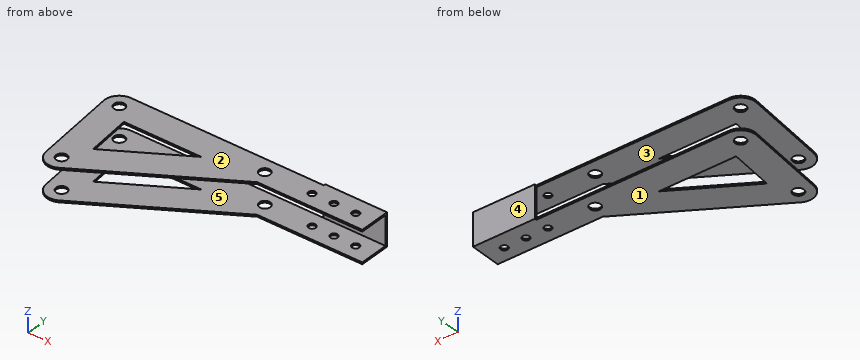
```python
from build123d import *

# Parameters (mm, degrees)
SKETCH_1_R      = 1.5
SKETCH_1_R_2    = 1
EXTRUDE_1_DEPTH = 0.5
SKETCH_2_R      = 1.5
SKETCH_2_R_2    = 1
EXTRUDE_2_DEPTH = 0.5
SKETCH_3_W      = 17
SKETCH_3_H      = 9
EXTRUDE_3_DEPTH = 0.5


with BuildPart() as part:
    # Sketch 1 → Extrude 1 (new body)
    with BuildSketch(Plane.XY):
        with BuildLine():
            Line((-6.593488685, 7.462066188), (63.406511315, 7.462066188))
            Line((63.406511315, 7.462066188), (63.406511315, -0.537933812))
            Line((63.406511315, -0.537933812), (34.527914712, -0.537933812))
            Line((34.527914712, -0.537933812), (-2.101613692, -22.82810419))
            ThreePointArc((-2.101613692, -22.82810419), (-5.955067108, -22.996117417), (-8.158923454, -19.830623953))
            Line((-8.158923454, -19.830623953), (-10.571423454, 3.04250097))
            ThreePointArc((-10.571423454, 3.04250097), (-9.566556198, 6.138046301), (-6.593488685, 7.462066188))
        make_face()
        with Locations((-6.593488685, 3.462066188)):
            Circle(SKETCH_1_R, mode=Mode.SUBTRACT)
        with Locations((33.406511315, 3.462066188)):
            Circle(SKETCH_1_R, mode=Mode.SUBTRACT)
        with Locations((-4.180988685, -19.411058735)):
            Circle(SKETCH_1_R, mode=Mode.SUBTRACT)
        with Locations((58.406511315, 3.462066188)):
            Circle(SKETCH_1_R_2, mode=Mode.SUBTRACT)
        with Locations((52.406511315, 3.462066188)):
            Circle(SKETCH_1_R_2, mode=Mode.SUBTRACT)
        with Locations((46.406511315, 3.462066188)):
            Circle(SKETCH_1_R_2, mode=Mode.SUBTRACT)
        Polygon((-2.149408554, -0.537933812), (19.138675105, -0.537933812), (-0.865471009, -12.711058735), align=None, mode=Mode.SUBTRACT)
    extrude(amount=EXTRUDE_1_DEPTH)



with BuildPart() as body_2:
    # Sketch 2 → Extrude 2 (new body)
    with BuildSketch(Plane.XY.offset(-8)):
        with BuildLine():
            Line((-2.101613692, -22.82810419), (34.527914712, -0.537933812))
            Line((34.527914712, -0.537933812), (63.406511315, -0.537933812))
            Line((63.406511315, -0.537933812), (63.406511315, 7.462066188))
            Line((63.406511315, 7.462066188), (-6.593488685, 7.462066188))
            ThreePointArc((-6.593488685, 7.462066188), (-9.566556198, 6.138046301), (-10.571423454, 3.04250097))
            Line((-10.571423454, 3.04250097), (-8.158923454, -19.830623953))
            ThreePointArc((-8.158923454, -19.830623953), (-5.955067108, -22.996117417), (-2.101613692, -22.82810419))
        make_face()
        with Locations((-4.180988685, -19.411058735)):
            Circle(SKETCH_2_R, mode=Mode.SUBTRACT)
        with Locations((33.406511315, 3.462066188)):
            Circle(SKETCH_2_R, mode=Mode.SUBTRACT)
        with Locations((-6.593488685, 3.462066188)):
            Circle(SKETCH_2_R, mode=Mode.SUBTRACT)
        with Locations((52.406511315, 3.462066188)):
            Circle(SKETCH_2_R_2, mode=Mode.SUBTRACT)
        with Locations((58.406511315, 3.462066188)):
            Circle(SKETCH_2_R_2, mode=Mode.SUBTRACT)
        with Locations((46.406511315, 3.462066188)):
            Circle(SKETCH_2_R_2, mode=Mode.SUBTRACT)
        Polygon((-0.865471009, -12.711058735), (19.138675105, -0.537933812), (-2.149408554, -0.537933812), align=None, mode=Mode.SUBTRACT)
    extrude(amount=-EXTRUDE_2_DEPTH)


with BuildPart() as part_1:
    add(part.part)

    add(body_2.part)  # Extrude 3 merges body 2
    # Sketch 3 → Extrude 3 (add)
    with BuildSketch(Plane(origin=(0, 7.462066188, 0), x_dir=(1, 0, 0), z_dir=(0, 1, 0))):
        with Locations((54.906511315, 4)):
            Rectangle(SKETCH_3_W, SKETCH_3_H)
    extrude(amount=EXTRUDE_3_DEPTH)


solid = part_1.part
```
Part model, mm, in its own coordinate system. Face numbers are marked on the shaded views. A direction names the side the tool comes from. Round coordinates to 2 decimals unless told otherwise and drop trailing zeros. Loops run counter-clockwise (first coordinate to the right, second up) from the corner with the lowest first, then second, coordinate; pieces in that order, holes last.
1. Slice it at A-A (y = -11.5). Give the cut face in (x, z).
Solutions:
outline: (-9.04, -8.5) - (-0.99, -8.5) - (-0.99, -8) - (-9.04, -8) - close; (-9.04, 0) - (-0.99, 0) - (-0.99, 0.5) - (-9.04, 0.5) - close; (1.12, -8.5) - (16.51, -8.5) - (16.51, -8) - (1.12, -8) - close; (1.12, 0) - (16.51, 0) - (16.51, 0.5) - (1.12, 0.5) - close
2. Drill centre lines: line 1 along Z through (x, y) = (55, 6.5); line 2 along Y through (x, z) = (50.5, -4.75). Where is each one in solid material? Low to high.
Solutions:
line 1: z = -8.5 to -8, 0 to 0.5
line 2: y = 7.46 to 7.96
3. Slice it at C-C (x = -3.5). Give the cut face in (y, z).
Solutions:
outline: (-23.35, -8.5) - (-20.75, -8.5) - (-20.75, -8) - (-23.35, -8) - close; (-23.35, 0) - (-20.75, 0) - (-20.75, 0.5) - (-23.35, 0.5) - close; (-18.07, -8.5) - (7.46, -8.5) - (7.46, -8) - (-18.07, -8) - close; (-18.07, 0) - (7.46, 0) - (7.46, 0.5) - (-18.07, 0.5) - close
4. Two-plate mould, pull along Z, no slides. Class the marked faces 1, 2 and 3: pulls with the +Z half, pulls with the -Z half, needs draft (parallel to the pull), parting line crosses it, or undercut.
Solutions:
face 1: pulls with the -Z half
face 2: pulls with the +Z half
face 3: undercut
5. 3-axis set-ups, long thin cutter, end or side, ignore diameter. For the marked faces 4 and 5: which of +Z, -Z, +X, -X, +Y, -Y reach the whole face in a straight line?
Solutions:
face 4: +Z, -Z, +X, -X, +Y
face 5: +X, -X, -Y
6. Flat gauge pins, fed straight in: pin 1 (1.5 mm diameter, centred on y = -8, z = -0.5, fed in from +X); pin 2 (2.5 mm diameter, centred on x = 54.5, z = -6, fed in from -Y); pin 3 (2.5 mm diameter, centred on x = -6.59, y = 3.46, fed in from +Z). Where does each tip first touch, or does it go through?
Solutions:
pin 1: stops at x = 23.18
pin 2: stops at y = 7.46
pin 3: passes through
7. Slice it at D-D (y = -17). Give the cut face in (x, z), and give its area (3 significant figures).
Solutions:
outline: (-8.46, -8.5) - (7.48, -8.5) - (7.48, -8) - (-8.46, -8) - close; (-8.46, 0) - (7.48, 0) - (7.48, 0.5) - (-8.46, 0.5) - close
area: 15.9 mm2
8. Slice it at B-B (x = 41). Give the cut face in (y, z), and give its area (3 significant figures).
Solutions:
outline: (-0.54, -8.5) - (7.46, -8.5) - (7.46, -8) - (-0.54, -8) - close; (-0.54, 0) - (7.46, 0) - (7.46, 0.5) - (-0.54, 0.5) - close
area: 8.00 mm2
